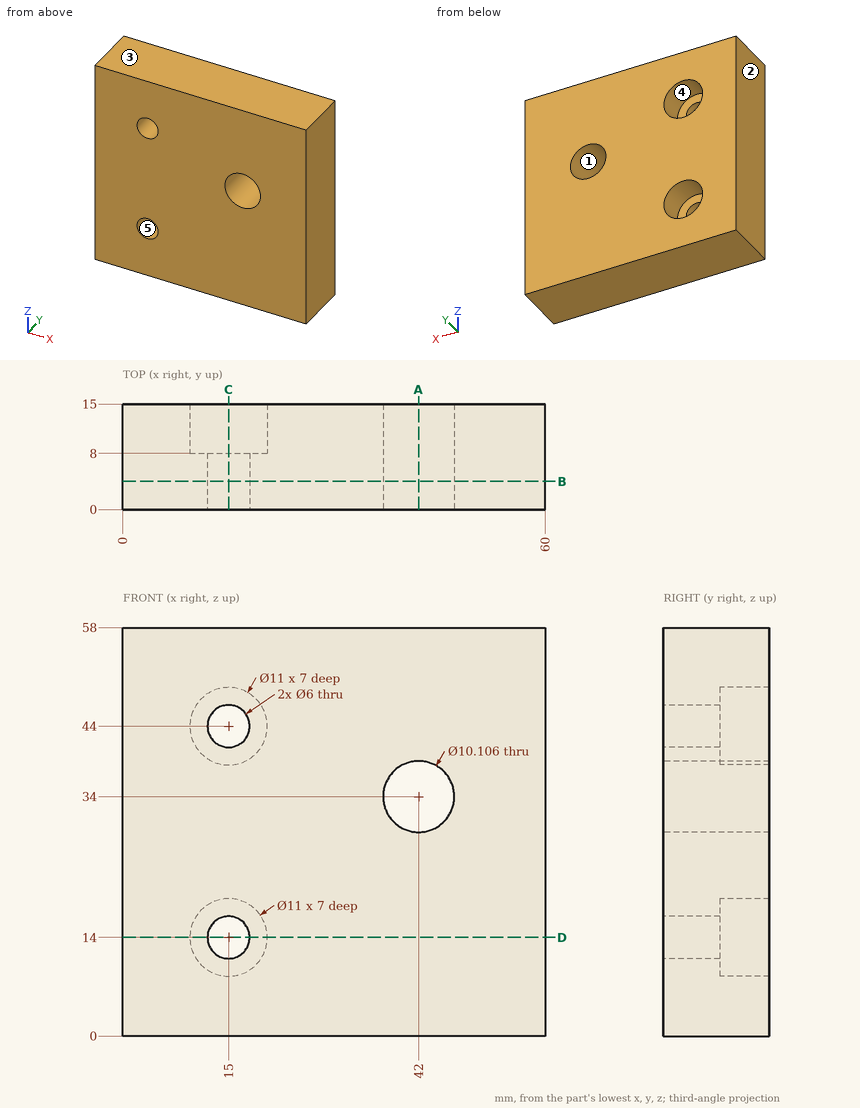
Geometry check sheet. Reference: drawing and pictorial views, mm from the part's lowest x, y, z. A direction names the side the tool comes from. Give positions to 0.01 mm unless a question says otherwise; leave off trailing zeros. Loops run counter-clockwise (first coordinate to the right, second up) from the corner with the lowest first, then second, coordinate; pieces in that order, holes last. Notation, with made-up numbers: M 76,72.5 L 93,72.5 A18 ccw 93,80.5 Z; hole C 51,-14.75 d4. An arc over 180 degrees is marked long. One line per question, with ' | ' between items.
Item 1: Section check C-C, the plane x = 15. Record the cut outline in (y, z), plus the area to 3 significant figures.
Completed:
outline: M 0,0 L 15,0 L 15,8.5 L 8,8.5 L 8,11 L 0,11 Z; M 0,17 L 8,17 L 8,19.5 L 15,19.5 L 15,38.5 L 8,38.5 L 8,41 L 0,41 Z; M 0,47 L 8,47 L 8,49.5 L 15,49.5 L 15,58 L 0,58 Z | area: 620 mm^2
Item 2: Tool access check on the marked faces 4 and 5. Record the directions out of +Z, -Z, +X, -X, +Y, -Y that give a thin tool (end or side, any length) a straight path to the whole face; none if there is none.
Completed:
face 4: +Y | face 5: +Y, -Y
Item 3: Section check A-A, the plane x = 42. Record the cut outline in (y, z), plus the area to 3 significant figures.
Completed:
outline: M 0,0 L 15,0 L 15,28.95 L 0,28.95 Z; M 0,39.05 L 15,39.05 L 15,58 L 0,58 Z | area: 718 mm^2
Item 4: Draft check along X on the marked faces 1, 2 and 3. Enter one of: +X half, -X half, draft (parallel to the pull), parting line (faces both ways), or undercut.
Completed:
face 1: undercut | face 2: -X half | face 3: draft
Item 5: Section check B-B, the plane y = 4. Record the cut outline in (x, z), plus the area to 3 significant figures.
Completed:
outline: M 0,0 L 60,0 L 60,58 L 0,58 Z; hole C 15,14 d6; hole C 15,44 d6; hole C 42,34 d10.11 | area: 3,340 mm^2
Item 6: Depth check by flat-ended pin: P1, Ø10, axis at x = 15, z = 14, coming from the +Y side. Enter the tip coordinate at first touch or a pass-through.
Completed:
P1: stops at y = 8
Item 7: Section check D-D, the plane z = 14. Record the cut outline in (x, y), plus the area to 3 significant figures.
Completed:
outline: M 0,0 L 12,0 L 12,8 L 9.5,8 L 9.5,15 L 0,15 Z; M 18,0 L 60,0 L 60,15 L 20.5,15 L 20.5,8 L 18,8 Z | area: 775 mm^2
Item 8: Thickness scan on line 1 (Z direction, x = 15, y = 4); line 2 (X direction, y = 6.5, z = 34); line 3 (Z direction, x = 14.5, y = 10). Record the ranges inside material, lowest first. Write a range as [from, to].
Completed:
line 1: z = [0, 11], [17, 41], [47, 58] | line 2: x = [0, 36.95], [47.05, 60] | line 3: z = [0, 8.52], [19.48, 38.52], [49.48, 58]
